For this review, take the finished solid that the model builds, in its own axes (mm). A direction names the side the tool comes from. Coordinates: 2 decimals unless noted, no trailing zeros. Loops run counter-clockwise (first coordinate to the right, second up) from the corner with the lowest first, then second, coordinate; pieces in that order, holes last. Notation, with made-up numbers: (-33, -22) -> (7, -22) arc R23 ccw to (7, 7) -> close; hole circle Ø3 at (80.25, -1.75). An arc over 180 degrees is marked (long way). Answer in a Markdown table with one row per item.
from build123d import *

# Parameters (mm, degrees)
F0_W     = 32
F0_H     = 32
F0_R     = 1.1
F0_R_2   = 7
F1_DEPTH = 2
F2_DEPTH = 24


with BuildPart() as f1:
    # F0 (on Front) → F1 (new body)
    with BuildSketch(Plane.XZ):
        Rectangle(F0_W, F0_H)
        with Locations((-14, -14)):
            Circle(F0_R, mode=Mode.SUBTRACT)
        with Locations((14, -14)):
            Circle(F0_R, mode=Mode.SUBTRACT)
        with Locations((-14, 14)):
            Circle(F0_R, mode=Mode.SUBTRACT)
        Circle(F0_R_2, mode=Mode.SUBTRACT)
        with Locations((14, 14)):
            Circle(F0_R, mode=Mode.SUBTRACT)
        Circle(F0_R_2)
    extrude(amount=F1_DEPTH)

    # F0 (on Front) → F2 (join)
    with BuildSketch(Plane.XZ):
        Circle(F0_R_2)
    extrude(amount=F2_DEPTH)


solid = f1.part
Item 1: Take a section at B-B, the plane z = 14. State the section outline as (x, y) points, and give its area (3 significant figures).
Worked answers:
| item | result |
|---|---|
| outline | (-16, -2) -> (-15.1, -2) -> (-15.1, 0) -> (-16, 0) -> close; (-12.9, -2) -> (12.9, -2) -> (12.9, 0) -> (-12.9, 0) -> close; (15.1, -2) -> (16, -2) -> (16, 0) -> (15.1, 0) -> close |
| area | 55.2 mm² |
Item 2: For L1, parallel to Z at x = 14, y = -0.8; L2, parallel to Y at x = -13.5, z = 7; L3, parallel to X at y = -5.25, z = -5, list the stretches that pass through material, from the lowest coordinate up.
Worked answers:
| item | result |
|---|---|
| L1 | -16 to -15.1, -12.9 to 12.9, 15.1 to 16 |
| L2 | -2 to 0 |
| L3 | -4.9 to 4.9 |
Item 3: Take a section at C-C, the plane z = 0. State the section outline as (x, y) points.
Worked answers:
| item | result |
|---|---|
| outline | (-16, -2) -> (-7, -2) -> (-7, -24) -> (7, -24) -> (7, -2) -> (16, -2) -> (16, 0) -> (-16, 0) -> close |
Item 4: Insertion check: pin 1 (6 mm diameter, centred on y = -6, z = -11.5, fed in from -X); pin 2 (1 mm diameter, centred on x = 10.5, z = 6.5, fed in from -Y); pin 3 (5 mm diameter, centred on x = 6.5, y = -18.5, fed in from -Z); pin 4 (3 mm diameter, centred on y = -15.5, z = 3.5, fed in from -X). Each pin has a flat end and moves straight along its axis. Give the tip position at first contact, or say it passes through.
Worked answers:
| item | result |
|---|---|
| pin 1 | through |
| pin 2 | y = -2 |
| pin 3 | z = -5.74 |
| pin 4 | x = -6.71 |
Item 5: Take a section at D-D, the plane x = 0. State the section outline as (y, z) points, and give its area (3 significant figures).
Worked answers:
| item | result |
|---|---|
| outline | (-24, -7) -> (-2, -7) -> (-2, -16) -> (0, -16) -> (0, 16) -> (-2, 16) -> (-2, 7) -> (-24, 7) -> close |
| area | 372 mm² |
Item 6: For faces 1 (the flat face through (0, -1, 16)), 2 (the cylindrical face through (6.466, -12.846, -2.681)), list the 3-axis set-ups (+Z, -Z, +X, -X, +Y, -Y) from which the entire face can be reached by the end or side of a thin tool; tool diameter is ignored.
Worked answers:
| item | result |
|---|---|
| face 1 | +Z, +X, -X, +Y, -Y |
| face 2 | -Y |
Item 7: Take a section at A-A, the plane x = 14. State the section outline as (y, z) points.
Worked answers:
| item | result |
|---|---|
| outline | (-2, -16) -> (0, -16) -> (0, -15.1) -> (-2, -15.1) -> close; (-2, -12.9) -> (0, -12.9) -> (0, 12.9) -> (-2, 12.9) -> close; (-2, 15.1) -> (0, 15.1) -> (0, 16) -> (-2, 16) -> close |
Item 8: The part is to be moulded in two halves that separate along Z. For faces 3 (the flat face through (0, -1, -16)), 4 (the flat face through (-0.2, -2, 7.3)), 5 (the cylindrical face through (-14.238, -0.986, 12.926)), say which applies: +Z half, -Z half, draft (parallel to the pull), parting line (faces both ways), or undercut.
Worked answers:
| item | result |
|---|---|
| face 3 | -Z half |
| face 4 | draft |
| face 5 | undercut |
